```python
from build123d import *

# Parameters (mm, degrees)
SKETCH_1_W               = 80
SKETCH_1_H               = 70
SKETCH_1_R               = 10
EXTRUDE_1_DEPTH          = 5
EXTRUDE_2_DEPTH          = 55
CUT_EXTRUDE_1_DEPTH      = 60
CUT_EXTRUDE_1_DEPTH_BACK = 60
SKETCH_3_R               = 12
SKETCH_3_R_2             = 1.5
FILLET_3_R               = 1.6
SKETCH_4_R               = 1.5
CUT_EXTRUDE_2_DEPTH      = 10
SKETCH_5_W               = 80
SKETCH_5_H               = 6
CUT_EXTRUDE_3_DEPTH      = 10
FILLET_4_R               = 10
CUT_EXTRUDE_4_DEPTH      = 10
FILLET_5_R               = 2
SKETCH_8_W               = 50
SKETCH_8_H               = 45
SKETCH_8_R               = 3.5
SKETCH_8_R_2             = 1.5
EXTRUDE_3_DEPTH          = 3
FILLET_6_R               = 10
SKETCH_10_R              = 12
SKETCH_10_R_2            = 1.5
SKETCH_10_R_3            = 3.5
EXTRUDE_4_DEPTH          = 5
SKETCH_12_R              = 12
SKETCH_12_R_2            = 10.5
EXTRUDE_5_DEPTH          = 4
SKETCH_13_R              = 21
SKETCH_13_R_2            = 12
EXTRUDE_6_DEPTH          = 2


with BuildPart() as part:
    # 草图1 → 凸台-拉伸1 (new body)
    with BuildSketch(Plane(origin=(0, 0, 0), x_dir=(1, 0, 0), z_dir=(0, 1, 0))):
        Rectangle(SKETCH_1_W, SKETCH_1_H)
        with Locations(Location((0, 0, 0), (0, 0, 270))):
            Circle(SKETCH_1_R, mode=Mode.SUBTRACT)
    extrude(amount=EXTRUDE_1_DEPTH)

    # 草图2 → 凸台-拉伸2 (add)
    with BuildSketch(Plane(origin=(0, 5, 0), x_dir=(1, 0, 0), z_dir=(0, 1, 0))):
        Polygon((-25, -9), (25, -9), (25, -20), (40, -20), (40, -25), (20.5, -25), (20.5, -13), (-20.5, -13), (-20.5, -25), (-40, -25), (-40, -20), (-25, -20), align=None)
    extrude(amount=EXTRUDE_2_DEPTH)

    # 草图3 → 切除-拉伸1 (cut, two sides: drawn at the far end of the back side and taken through both)
    with BuildSketch(Plane.XY.offset(13).offset(-CUT_EXTRUDE_1_DEPTH_BACK)):
        with Locations((0, 26.15)):
            Circle(SKETCH_3_R)
        with Locations((15.5, 41.65)):
            Circle(SKETCH_3_R_2)
        with Locations((15.5, 10.65)):
            Circle(SKETCH_3_R_2)
        with Locations((-15.5, 10.65)):
            Circle(SKETCH_3_R_2)
        with Locations((-15.5, 41.65)):
            Circle(SKETCH_3_R_2)
        with Locations((-30, 13)):
            Circle(SKETCH_3_R_2)
        with Locations((-30, 33)):
            Circle(SKETCH_3_R_2)
        with Locations((-30, 53)):
            Circle(SKETCH_3_R_2)
        with Locations((30, 53)):
            Circle(SKETCH_3_R_2)
        with Locations((30, 33)):
            Circle(SKETCH_3_R_2)
        with Locations((30, 13)):
            Circle(SKETCH_3_R_2)
    extrude(amount=CUT_EXTRUDE_1_DEPTH + CUT_EXTRUDE_1_DEPTH_BACK, mode=Mode.SUBTRACT)

    # 圆角3
    fillet_3_edges = [part.edges().sort_by_distance(p)[0] for p in [
        (25, 32.5, 20),
        (25, 32.5, 9),
        (-25, 32.5, 9),
        (-25, 32.5, 20),
        (-20.5, 32.5, 25),
        (-20.5, 32.5, 13),
        (20.5, 32.5, 13),
        (20.5, 32.5, 25),
    ]]
    fillet(fillet_3_edges, radius=FILLET_3_R)

    # 草图4 → 切除-拉伸2 (cut)
    with BuildSketch(Plane(origin=(0, 5, 0), x_dir=(1, 0, 0), z_dir=(0, 1, 0))):
        with Locations(Location((30, 14, 0), (0, 0, 270))):
            Circle(SKETCH_4_R)
        with Locations(Location((30, -6, 0), (0, 0, 270))):
            Circle(SKETCH_4_R)
        with Locations(Location((-30, -6, 0), (0, 0, 90))):
            Circle(SKETCH_4_R)
        with Locations(Location((-30, 14, 0), (0, 0, 90))):
            Circle(SKETCH_4_R)
    extrude(amount=-CUT_EXTRUDE_2_DEPTH, mode=Mode.SUBTRACT)

    # 草图5 → 切除-拉伸3 (cut)
    with BuildSketch(Plane(origin=(0, 5, 0), x_dir=(1, 0, 0), z_dir=(0, 1, 0))):
        with Locations((0, 32)):
            Rectangle(SKETCH_5_W, SKETCH_5_H)
    extrude(amount=-CUT_EXTRUDE_3_DEPTH, mode=Mode.SUBTRACT)

    # 圆角4
    fillet_4_edges = [part.edges().sort_by_distance(p)[0] for p in [
        (-40, 2.5, -29),
        (40, 2.5, -29),
        (40, 2.5, 35),
        (-40, 2.5, 35),
    ]]
    fillet(fillet_4_edges, radius=FILLET_4_R)

    # 草图6 → 切除-拉伸4 (cut)
    with BuildSketch(Plane.XY.offset(13)):
        Polygon((0, 5), (5, 5), (5, 10), (-5, 10), (-5, 5), align=None)
    extrude(amount=-CUT_EXTRUDE_4_DEPTH, mode=Mode.SUBTRACT)

    # 圆角5
    # the kernel refuses this fillet: 2 mm, written as the material it adds along each edge
    with BuildSketch(Plane(origin=(-5, 5, 13), x_dir=(1, 0, 0), z_dir=(0, 0, -1))) as fillet_5_piece_1_section:
        with BuildLine():
            CenterArc((FILLET_5_R, -FILLET_5_R), FILLET_5_R, 90, 90)
            Line((0, -FILLET_5_R), (0, 0))
            Line((0, 0), (FILLET_5_R, 0))
        make_face()
    fillet_5_piece_1 = extrude(amount=4, mode=Mode.PRIVATE)
    fillet_5_piece_1 = fillet_5_piece_1 - Plane(origin=(0, 5.457543307, 0), x_dir=(0, 0, 1), z_dir=(0, -1, 0)) * Cylinder(10, 17, mode=Mode.PRIVATE)
    add(fillet_5_piece_1)
    with BuildSketch(Plane(origin=(-5, 10, 13), x_dir=(0, -1, 0), z_dir=(0, 0, -1)), Plane(origin=(5, 10, 13), x_dir=(-1, 0, 0), z_dir=(0, 0, -1))) as fillet_5_piece_2:
        with BuildLine():
            CenterArc((FILLET_5_R, -FILLET_5_R), FILLET_5_R, 90, 90)
            Line((0, -FILLET_5_R), (0, 0))
            Line((0, 0), (FILLET_5_R, 0))
        make_face()
    extrude(amount=4)
    with BuildSketch(Plane(origin=(5, 5, 13), x_dir=(-1, 0, 0), z_dir=(0, 0, -1))) as fillet_5_piece_3_section:
        with BuildLine():
            CenterArc((FILLET_5_R, FILLET_5_R), FILLET_5_R, 180, 90)
            Line((0, FILLET_5_R), (0, 0))
            Line((0, 0), (FILLET_5_R, 0))
        make_face()
    fillet_5_piece_3 = extrude(amount=4, mode=Mode.PRIVATE)
    fillet_5_piece_3 = fillet_5_piece_3 - Plane(origin=(0, 5.457543307, 0), x_dir=(0, 0, 1), z_dir=(0, -1, 0)) * Cylinder(10, 17, mode=Mode.PRIVATE)
    add(fillet_5_piece_3)

    # 草图8 → 凸台-拉伸3 (add)
    with BuildSketch(Plane.XZ):
        Rectangle(SKETCH_8_W, SKETCH_8_H)
        with Locations(Location((0, 0, 0), (0, 0, 270))):
            Circle(SKETCH_8_R, mode=Mode.SUBTRACT)
        with Locations(Location((0, 7, 0), (0, 0, 270))):
            Circle(SKETCH_8_R_2, mode=Mode.SUBTRACT)
        with Locations(Location((7, 0, 0), (0, 0, 270))):
            Circle(SKETCH_8_R_2, mode=Mode.SUBTRACT)
        with Locations(Location((-7, 0, 0), (0, 0, 90))):
            Circle(SKETCH_8_R_2, mode=Mode.SUBTRACT)
        with Locations(Location((0, -7, 0), (0, 0, 90))):
            Circle(SKETCH_8_R_2, mode=Mode.SUBTRACT)
    extrude(amount=EXTRUDE_3_DEPTH)

    # 圆角6
    fillet_6_edges = [part.edges().sort_by_distance(p)[0] for p in [
        (25, -1.5, -22.5),
        (25, -1.5, 22.5),
        (-25, -1.5, 22.5),
        (-25, -1.5, -22.5),
    ]]
    fillet(fillet_6_edges, radius=FILLET_6_R)

    # 草图10 → 凸台-拉伸4 (add)
    with BuildSketch(Plane.XZ.offset(3)):
        with Locations(Location((0, 0, 0), (0, 0, 270))):
            Circle(SKETCH_10_R)
        with Locations(Location((0, -7, 0), (0, 0, 90))):
            Circle(SKETCH_10_R_2, mode=Mode.SUBTRACT)
        with Locations(Location((-7, 0, 0), (0, 0, 90))):
            Circle(SKETCH_10_R_2, mode=Mode.SUBTRACT)
        with Locations(Location((7, 0, 0), (0, 0, 270))):
            Circle(SKETCH_10_R_2, mode=Mode.SUBTRACT)
        with Locations(Location((0, 0, 0), (0, 0, 270))):
            Circle(SKETCH_10_R_3, mode=Mode.SUBTRACT)
        with Locations(Location((0, 7, 0), (0, 0, 270))):
            Circle(SKETCH_10_R_2, mode=Mode.SUBTRACT)
    extrude(amount=EXTRUDE_4_DEPTH)

    # 草图12 → 凸台-拉伸5 (add)
    with BuildSketch(Plane.XZ.offset(8)):
        with Locations(Location((0, 0, 0), (0, 0, 270))):
            Circle(SKETCH_12_R)
        with Locations(Location((0, 0, 0), (0, 0, 270))):
            Circle(SKETCH_12_R_2, mode=Mode.SUBTRACT)
    extrude(amount=EXTRUDE_5_DEPTH)

    # 草图13 → 凸台-拉伸6 (add)
    with BuildSketch(Plane.XZ.offset(3)):
        with Locations(Location((0, 0, 0), (0, 0, 90))):
            Circle(SKETCH_13_R)
        with Locations(Location((0, 0, 0), (0, 0, 270))):
            Circle(SKETCH_13_R_2, mode=Mode.SUBTRACT)
    extrude(amount=EXTRUDE_6_DEPTH)


solid = part.part
```
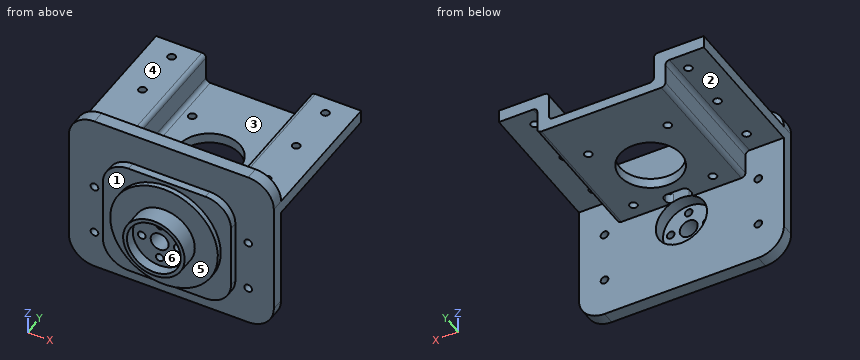
Design review of the part built by this model. Coordinates are the model's own, in mm. Face numbers are marked on the shaded views. A direction names the side the tool comes from. Give positions to 0.01 mm unless a question says otherwise; leave off trailing zeros. Order: outer loops, then holes, each group sorted by start corner. A loop starts at its lowest first (then second) coordinate and runs counter-clockwise, first axis right, second up. Notation, with made-up numbers: (42, 37.25) -> (92, 37.25) arc R27 ccw to (92, 74.25) -> close; hole circle Ø6 at (39.5, 8.5). An arc over 180 degrees is marked (long way). Write item = value, one per line. Start each with the question number.
(1) We need section D-D on x = 0. State how many separate pieces and enclosed holes the cut face has, plus the area to 3 significant figures.
(2) For pin 1 (3 mm diameter, centred on x = -8, z = 27.5, fed in from +Y); pin 2 (2 mm diameter, centred on x = 12.5, y = -1.5, fed in from +Z); pin 3 (3.5 mm diameter, centred on x = 30, y = 33, fed in from +Z), all flat-tipped, find the tip position at first contact; note any pin that passes through.
(3) We need section A-A on y = 1.5. Write out the cut boundary in (x, z).
(4) Mouldability with a two-part tool opening along X and no side actions: class the marked faces 5 and 6 as +X half, -X half, draft (parallel to the pull), parting line (faces both ways), or undercut.
(5) To check wall thickness, follow line 1 along X through (y, z) = (2.4, -14); line 2 along Y through (x, z) = (-30, 23.9); line 3 along X through (y, z) = (-6.25, 0). State the ranges of each line that lie inside material, in increasing order.
(6) We need section B-B on z = -14. Write out the cut boundary in (x, y).
(7) For the marked faces 1, 2, 3 and 4, list the 3-axis set-ups (+Z, -Z, +X, -X, +Y, -Y) from which the entire face can be reached by the end or side of a thin tool; tool diameter is ignored.
(8) We need section C-C on y = 22. Write out the cut boundary in (x, z).
Numbers:
q1.separate_pieces = 6
q1.enclosed_holes = 0
q1.area = 523 mm^2
q2.pin_1 = 5
q2.pin_2 = 22.5
q2.pin_3 = 25
q3.outline = (-40, -19) arc R10 ccw to (-30, -29) -> (30, -29) arc R10 ccw to (40, -19) -> (40, 25) arc R10 ccw to (30, 35) -> (-30, 35) arc R10 ccw to (-40, 25) -> close; hole circle Ø3 at (-30, -14); hole circle Ø3 at (-30, 6); hole circle Ø20 at (0, 0); hole circle Ø3 at (30, -14); hole circle Ø3 at (30, 6)
q4.face_5 = draft
q4.face_6 = undercut
q5.line_1 = -40 to -31.5, -28.5 to 28.5, 31.5 to 40
q5.line_2 = 0 to 11.5, 14.5 to 31.5, 34.5 to 51.5, 54.5 to 60
q5.line_3 = -12 to -8.5, -5.5 to -3.5, 3.5 to 5.5, 8.5 to 12
q6.outline = (-40, 0) -> (-31.5, 0) -> (-31.5, 5) -> (-40, 5) -> close; (-28.5, 0) -> (-24.89, 0) -> (-24.89, -3) -> (-15.65, -3) -> (-15.65, -5) -> (15.65, -5) -> (15.65, -3) -> (24.89, -3) -> (24.89, 0) -> (28.5, 0) -> (28.5, 5) -> (-28.5, 5) -> close; (31.5, 0) -> (40, 0) -> (40, 5) -> (31.5, 5) -> close
q7.face_1 = -Y
q7.face_2 = -Z, -X, +Y
q7.face_3 = +Z, +Y
q7.face_4 = +Z, +X, -X, +Y
q8.outline = (-40, 20) -> (-26.6, 20) arc R1.6 cw to (-25, 18.4) -> (-25, 10.6) arc R1.6 ccw to (-23.4, 9) -> (-11.26, 9) -> (-11.26, 13) -> (-18.9, 13) arc R1.6 cw to (-20.5, 14.6) -> (-20.5, 23.4) arc R1.6 ccw to (-22.1, 25) -> (-40, 25) -> close; (11.26, 9) -> (23.4, 9) arc R1.6 ccw to (25, 10.6) -> (25, 18.4) arc R1.6 cw to (26.6, 20) -> (40, 20) -> (40, 25) -> (22.1, 25) arc R1.6 ccw to (20.5, 23.4) -> (20.5, 14.6) arc R1.6 cw to (18.9, 13) -> (11.26, 13) -> close
